Autodesk Inventor part; units mm, degrees
ref_plane "YZ Plane" through (0, 0, 0) normal (1, 0, 0) x (0, 1, 0)
ref_plane "XZ Plane" through (0, 0, 0) normal (0, 1, 0) x (-1, 0, 0)
ref_plane "XY Plane" through (0, 0, 0) normal (0, 0, 1) x (1, 0, 0)
sketch "Sketch3" plane through (0, 0, 0) normal (0, 0, 1) x (1, 0, 0)
  line L0 (0, -119) -> (0, 119)
  line L1 (-189, 0) -> (189, 0)
  line L2 (-135, -85) -> (135, -85)
  line L3 (135, -85) -> (135, 85)
  line L4 (135, 85) -> (-135, 85)
  line L5 (-135, 85) -> (-135, -85)
  line L6 (-135, -85) -> (135, 85) construction
  line L7 (135, -85) -> (-135, 85) construction
  line L8 (-130, -80) -> (130, -80)
  line L9 (130, -80) -> (130, 80)
  line L10 (130, 80) -> (-130, 80)
  line L11 (-130, 80) -> (-130, -80)
  line L12 (-130, -80) -> (130, 80) construction
  line L13 (130, -80) -> (-130, 80) construction
  point P0 (0, 0)
  dimension "d0" = 270
  dimension "d1" = 170
  dimension "d2" = 260
  dimension "d3" = 160
extrude "Extrusion1" add sketch "Sketch3" along normal blind 85 contours L2 L5 L1 L11 L8 L0 | L0 L8 L9 L1 L3 L2 | L5 L4 L0 L10 L11 L1 | L1 L9 L10 L0 L4 L3
extrude "Extrusion2" add sketch "Sketch3" along normal blind 5 contours L8 L11 L1 L0 | L0 L1 L9 L8 | L1 L11 L10 L0 | L0 L10 L9 L1
fillet "Fillet1" radius 2 8 edges at (135, -85, 42.5) (135, 85, 42.5) (-135, 85, 42.5) (-135, -85, 42.5) (-135, 0, 0) (0, 85, 0) (0, -85, 0) (135, 0, 0)
equation "\"BendRadius\" = Thickness"
equation "\"BendReliefWidth\" = Thickness"
equation "\"BendReliefDepth\" = 0.5 * Thickness"
equation "\"CornerReliefSize\" = 4 * Thickness"
equation "\"MinimumRemnant\" = 2 * Thickness"
equation "\"TransitionRadius\" = BendRadius"
equation "\"JacobiRadiusSize\" = BendRadius"
equation "\"GapSize\" = Thickness"
properties part number "Batterybox"
The listing builds one solid part. Answer for the finished solid, in the listing's coordinates (mm). A direction names the side the tool comes from. Round coordinates to 2 decimals unless told otherwise and drop trailing zeros. Loops run counter-clockwise (first coordinate to the right, second up) from the corner with the lowest first, then second, coordinate; pieces in that order, holes last. Notation, with made-up numbers: M 18,76 L 65,76 A26 ccw 65,105 Z; hole C -40,66 d9. An arc over 180 degrees is marked long. Write each question's results on one line, items separated by ' | '. Start each with the question number.
1) Find section C-C on y = -20. Write down the section's boundary in (x, z).
2) Find section B-B on x = -34.5. Write down the section's boundary in (y, z), plus the area to 3 significant figures.
3) Which of the six approach directions +Z, -Z, +X, -X, +Y, -Y give full straight-line access (tool end or side, diameter ignored) to faces 5 (the flat face through (-2, 1, 0)), 6 (the flat face through (-2, -80, 44))?
4) Straight lines are drawn through the part: probe 1 along Y at (x, z) = (42.5, 7); probe 2 along X at (y, z) = (-2, 39); probe 3 along Z at (x, y) = (-64.5, -71). For each, find the intervals that lie inside material, in ascending order.
5) This flat-tipped pin is pushed along its axis until it touches: pin 1 (4 mm diameter, centred on x = -63.5, y = -56, fed in from +Z). Where does it stop, or does it pass through?
6) Determine the mould class of faces 1 (the flat face through (-135, 1, 43)), 2 (the flat face through (-2, 1, 5)), 3 (the flat face through (-130, 1, 44)), 4 (the flat face through (2, 85, 43)) for opening direction Y: pulls with the +Y half, pulls with the -Y half, needs draft (parallel to the pull), parting line crosses it, or undercut.
7) Find section A-A on z = 10. Write down the section's boundary in (x, y), plus the area to 3 significant figures.
Final values:
1) outline: M -135,2 A2 ccw -133,0 L 133,0 A2 ccw 135,2 L 135,85 L 130,85 L 130,5 L -130,5 L -130,85 L -135,85 Z
2) outline: M -85,2 A2 ccw -83,0 L 83,0 A2 ccw 85,2 L 85,85 L 80,85 L 80,5 L -80,5 L -80,85 L -85,85 Z | area: 1,650 mm²
3) face 5: -Z, +X, -X, +Y, -Y | face 6: +Z
4) probe 1: -85 to -80, 80 to 85 | probe 2: -135 to -130, 130 to 135 | probe 3: 0 to 5
5) pin 1: z = 5
6) face 1: needs draft | face 2: undercut | face 3: undercut | face 4: pulls with the +Y half
7) outline: M -135,-83 A2 ccw -133,-85 L 133,-85 A2 ccw 135,-83 L 135,83 A2 ccw 133,85 L -133,85 A2 ccw -135,83 Z; hole M -130,-80 L 130,-80 L 130,80 L -130,80 Z | area: 4,300 mm²
